The listing builds one solid part. Answer for the finished solid, in the listing's coordinates (mm). A direction names the side the tool comes from. Coordinates: 2 decimals unless noted, no trailing zeros. Order: outer loops, then holes, each group sorted by start corner. A loop starts at its lowest first (then second) coordinate and runs counter-clockwise, first axis right, second up. Notation, with made-up numbers: (-37.75, 62.25) -> (8.25, 62.25) arc R23 cw to (8.25, 97.25) -> close; hole circle Ø8 at (85, 41.25). An arc over 180 degrees is marked (long way). Write each question's results on one line, items separated by ' | '. Start each with the question number.
(1) The part is cut by section D-D, the plane z = 3. Give the vertices of the cut face in (x, y), then the cut area to 3 significant figures.
(2) The part is cut by section A-A, the plane y = 35. Give the vertices of the cut face in (x, z).
(3) A tool of negligible diameter and unlimited length cuts with its end or side. For faces 1 (the face through (31, 25, 3)), 2 (the face through (20.3, 38.05, -0.4)), 3 (the face through (15, 20, 0)), 4 (the face through (10, 0, 3)), from which of +Z, -Z, +X, -X, +Y, -Y can it reach the whole face along a straight path? Write none if from no direction.
(4) Given pin 1 (4.5 mm diameter, centred on x = 30, y = 35, fed in from -Z); pin 2 (2 mm diameter, centred on x = 33.5, z = 5.5, fed in from -Y); pin 3 (3.5 mm diameter, centred on y = 7.5, z = 2, fed in from +X); pin 4 (0.7 mm diameter, centred on x = 26, z = -0.5, fed in from +Y), each flat-ended and moving along its own axis, determine where each tip first touches the part or whether it passes through.
(5) The part is cut by section B-B, the plane x = 30. Give the vertices of the cut face in (y, z), then the cut area to 3 significant figures.
(6) The part is cut by section C-C, the plane y = 15. Give the vertices of the cut face in (x, z), then the cut area to 3 significant figures.
(7) Straight lines are drawn through the part: L1, parallel to Y at x = 10, z = 2; L2, parallel to Y at x = 30, z = -0.55; L3, parallel to X at y = 37, z = 0.75. For each, find the intervals that lie inside material, in ascending order.
```python
from build123d import *

# Parameters (mm, degrees)
SKETCH1_R           = 2.5
SKETCH1_R_2         = 1.1
BOSS_EXTRUDE1_DEPTH = 7
SKETCH2_W           = 0.9
SKETCH2_H           = 6.1
BOSS_EXTRUDE2_DEPTH = 40
CUT_EXTRUDE1_REACH  = 2.9
SKETCH3_R           = 2.5


with BuildPart() as part:
    # Sketch1 → Boss-Extrude1 (new body)
    with BuildSketch(Plane.XY):
        with BuildLine():
            Line((3, 0), (17, 0))
            ThreePointArc((17, 0), (19.121320344, 0.878679656), (20, 3))
            Line((20, 3), (20, 19))
            ThreePointArc((20, 19), (21.757359313, 23.242640687), (26, 25))
            Line((26, 25), (37, 25))
            ThreePointArc((37, 25), (39.121320344, 25.878679656), (40, 28))
            Line((40, 28), (40, 41))
            ThreePointArc((40, 41), (39.121320344, 43.121320344), (37, 44))
            Line((37, 44), (3, 44))
            ThreePointArc((3, 44), (0.878679656, 43.121320344), (0, 41))
            Line((0, 41), (0, 3))
            ThreePointArc((0, 3), (0.878679656, 0.878679656), (3, 0))
        make_face()
        with Locations((10, 35)):
            Circle(SKETCH1_R, mode=Mode.SUBTRACT)
        with Locations((30, 35)):
            Circle(SKETCH1_R, mode=Mode.SUBTRACT)
        with Locations((10, 5.4)):
            Circle(SKETCH1_R_2, mode=Mode.SUBTRACT)
        with Locations((10, 15)):
            Circle(SKETCH1_R_2, mode=Mode.SUBTRACT)
    extrude(amount=BOSS_EXTRUDE1_DEPTH)

    # Sketch2 → Boss-Extrude2 (add)
    with BuildSketch(Plane(origin=(40, 0, 0), x_dir=(0, 0, -1), z_dir=(1, 0, 0))):
        with Locations((0.45, 35)):
            Rectangle(SKETCH2_W, SKETCH2_H)
    extrude(amount=-BOSS_EXTRUDE2_DEPTH)

    # Sketch3 → Cut-Extrude1 (cut, up to next)
    with BuildSketch(Plane.XY, mode=Mode.PRIVATE) as cut_extrude1_sk1:
        with Locations((10, 35)):
            Circle(SKETCH3_R)
    cut_extrude1_tool1 = extrude(cut_extrude1_sk1.sketch, amount=-CUT_EXTRUDE1_REACH, mode=Mode.PRIVATE) & part.part
    add(cut_extrude1_tool1.solids().sort_by_distance((10, 35, 0))[0], mode=Mode.SUBTRACT)
    # Sketch3 → Cut-Extrude1 (cut, up to next)
    with BuildSketch(Plane.XY, mode=Mode.PRIVATE) as cut_extrude1_sk2:
        with Locations((30, 35)):
            Circle(SKETCH3_R)
    cut_extrude1_tool2 = extrude(cut_extrude1_sk2.sketch, amount=-CUT_EXTRUDE1_REACH, mode=Mode.PRIVATE) & part.part
    add(cut_extrude1_tool2.solids().sort_by_distance((30, 35, 0))[0], mode=Mode.SUBTRACT)


solid = part.part
```
Established:
1) outline: (0, 3) arc R3 ccw to (3, 0) -> (17, 0) arc R3 ccw to (20, 3) -> (20, 19) arc R6 cw to (26, 25) -> (37, 25) arc R3 ccw to (40, 28) -> (40, 41) arc R3 ccw to (37, 44) -> (3, 44) arc R3 ccw to (0, 41) -> close; hole circle Ø5 at (10, 35); hole circle Ø2.2 at (10, 5.4); hole circle Ø2.2 at (10, 15); hole circle Ø5 at (30, 35) | area: 1,210 mm^2
2) outline: (0, -0.9) -> (7.5, -0.9) -> (7.5, 7) -> (0, 7) -> close; (12.5, -0.9) -> (27.5, -0.9) -> (27.5, 7) -> (12.5, 7) -> close; (32.5, -0.9) -> (40, -0.9) -> (40, 7) -> (32.5, 7) -> close
3) face 1: +Z, -Z, +X, -Y | face 2: -Z, +X, -X, +Y | face 3: -Z, +X, -X, -Y | face 4: +Z, -Z, +X, -X, -Y
4) pin 1: passes through | pin 2: stops at y = 25 | pin 3: stops at x = 20 | pin 4: stops at y = 38.05
5) outline: (25, 0) -> (31.95, 0) -> (31.95, -0.9) -> (32.5, -0.9) -> (32.5, 7) -> (25, 7) -> close; (37.5, -0.9) -> (38.05, -0.9) -> (38.05, 0) -> (44, 0) -> (44, 7) -> (37.5, 7) -> close | area: 99.0 mm^2
6) outline: (0, 0) -> (8.9, 0) -> (8.9, 7) -> (0, 7) -> close; (11.1, 0) -> (20, 0) -> (20, 7) -> (11.1, 7) -> close | area: 125 mm^2
7) L1: y = 0 to 4.3, 6.5 to 13.9, 16.1 to 32.5, 37.5 to 44 | L2: y = 31.95 to 32.5, 37.5 to 38.05 | L3: x = 0 to 8.5, 11.5 to 28.5, 31.5 to 40
